For this review, take the finished solid that the model builds, in its own axes (mm). A direction names the side the tool comes from. Coordinates: 2 decimals unless noted, no trailing zeros. Order: outer loops, then holes, each group sorted by start corner. A loop starts at its lowest first (then second) coordinate and runs counter-clockwise, first axis right, second up. Notation, with made-up numbers: (40, 39.5) -> (80, 39.5) arc R14 ccw to (80, 55.5) -> close; hole circle Ø7 at (50.5, 52). An arc over 180 degrees is marked (long way). Answer as a JSON object with one key per item and string values. Group by question number.
1) Add section B-B, the plane x = -8. Write out the cut boundary in (y, z).
2) For pin 1 (0.8 mm diameter, centred on y = -3.5, z = 13, fed in from +X); pin 2 (4 mm diameter, centred on x = -8.5, y = -6, fed in from -Z); pin 3 (1 mm diameter, centred on x = 15, y = 2.5, fed in from -Z); pin 4 (1 mm diameter, centred on y = -1, z = 4.5, fed in from +X), all flat-tipped, find the tip position at first contact; note any pin that passes through.
3) Draft analysis for pull direction X (two halves, no side actions). For faces 6 (the flat face through (-23, 3, 4)), 7 (the flat face through (0, 3, 0)), 8 (the flat face through (-19.05, -4, -13)), state which applies: +X half, -X half, draft (parallel to the pull), parting line (faces both ways), or undercut.
4) Add section C-C, the plane y = 2.5. Write out the cut boundary in (x, z), then the cut area to 3 significant figures.
5) Wall thickness on L1, parallel to Z at x = 15, y = -2.5; L2, parallel to Y at x = 16.5, z = 3; L3, parallel to Y at x = -19, z = -7.5: over which ranges is each line inside the solid? List them lowest first.
6) Machinability: for faces 1 (the flat face through (13, 3, -9)), 2 (the flat face through (0, -4, 11.45)), 3 (the flat face through (-23, 3, -4)), 4 (the flat face through (-19.05, -4, 13)), 5 (the flat face through (19.05, -4, 13)), which of the approach directions +Z, -Z, +X, -X, +Y, -Y give a long, thin tool a straight path to every point of the face, cutting with its end or side? Answer none if there is none.
7) Add section A-A, the plane y = -2.25. Write out the cut boundary in (x, z).
8) Add section D-D, the plane z = 3. Write out the cut boundary in (x, y).
from build123d import *

# Parameters (mm, degrees)
SKETCH1_W          = 51
SKETCH1_H          = 28
BOARD_DEPTH        = 1.6
WROOM_MODULE_START = 1.6
SKETCH2_W          = 25.5
SKETCH2_H          = 18
WROOM_MODULE_DEPTH = 3.2
MICRO_USB_START    = 1.6
SKETCH3_W          = 6
SKETCH3_H          = 8
MICRO_USB_DEPTH    = 3
HEADER_A_START     = -8.5
SKETCH4_W          = 38.1
SKETCH4_H          = 2.5
HEADER_A_DEPTH     = 8.5
HEADER_B_START     = -8.5
SKETCH5_W          = 38.1
SKETCH5_H          = 2.5
HEADER_B_DEPTH     = 8.5


with BuildPart() as part:
    # Sketch1 → Board (new body)
    with BuildSketch(Plane(origin=(0, 0, 0), x_dir=(1, 0, 0), z_dir=(0, 1, 0))):
        Rectangle(SKETCH1_W, SKETCH1_H)
    extrude(amount=BOARD_DEPTH)

    # Sketch2 → WROOM_Module (add)
    with BuildSketch(Plane(origin=(0, 0, 0), x_dir=(1, 0, 0), z_dir=(0, 1, 0)).offset(WROOM_MODULE_START)):
        with Locations((12.75, 0)):
            Rectangle(SKETCH2_W, SKETCH2_H)
    extrude(amount=WROOM_MODULE_DEPTH)

    # Sketch3 → Micro_USB (add)
    with BuildSketch(Plane(origin=(0, 0, 0), x_dir=(1, 0, 0), z_dir=(0, 1, 0)).offset(MICRO_USB_START)):
        with Locations((-22.5, 0)):
            Rectangle(SKETCH3_W, SKETCH3_H)
    extrude(amount=MICRO_USB_DEPTH)

    # Sketch4 → Header_A (add)
    with BuildSketch(Plane(origin=(0, 0, 0), x_dir=(1, 0, 0), z_dir=(0, 1, 0)).offset(HEADER_A_START)):
        with Locations((0, 12.7)):
            Rectangle(SKETCH4_W, SKETCH4_H)
    extrude(amount=HEADER_A_DEPTH)

    # Sketch5 → Header_B (add)
    with BuildSketch(Plane(origin=(0, 0, 0), x_dir=(1, 0, 0), z_dir=(0, 1, 0)).offset(HEADER_B_START)):
        with Locations((0, -12.7)):
            Rectangle(SKETCH5_W, SKETCH5_H)
    extrude(amount=HEADER_B_DEPTH)


solid = part.part
Output values:
{
 "1": {"outline": "(-8.5, -13.95) -> (0, -13.95) -> (0, -14) -> (1.6, -14) -> (1.6, 14) -> (0, 14) -> (0, 13.95) -> (-8.5, 13.95) -> (-8.5, 11.45) -> (0, 11.45) -> (0, -11.45) -> (-8.5, -11.45) -> close"},
 "2": {"pin 1": "stops at x = 19.05", "pin 2": "stops at z = -13.95", "pin 3": "stops at z = -9", "pin 4": "passes through"},
 "3": {"face 6": "draft", "face 7": "undercut", "face 8": "-X half"},
 "4": {"outline": "(-25.5, -4) -> (-19.5, -4) -> (-19.5, 4) -> (-25.5, 4) -> close; (0, -9) -> (25.5, -9) -> (25.5, 9) -> (0, 9) -> close", "area": "507 mm²"},
 "5": {"L1": "z = -13.95 to -11.45, 11.45 to 13.95", "L2": "y = 0 to 4.8", "L3": "y = 0 to 1.6"},
 "6": {"face 1": "-Z, +X, -X, +Y", "face 2": "+X, -X, -Y", "face 3": "-Z, -X, +Y", "face 4": "+Z, -Z, -X, -Y", "face 5": "+Z, -Z, +X, -Y"},
 "7": {"outline": "(-19.05, -13.95) -> (19.05, -13.95) -> (19.05, -11.45) -> (-19.05, -11.45) -> close; (-19.05, 11.45) -> (19.05, 11.45) -> (19.05, 13.95) -> (-19.05, 13.95) -> close"},
 "8": {"outline": "(-25.5, 0) -> (25.5, 0) -> (25.5, 4.8) -> (0, 4.8) -> (0, 1.6) -> (-19.5, 1.6) -> (-19.5, 4.6) -> (-25.5, 4.6) -> close"}
}
